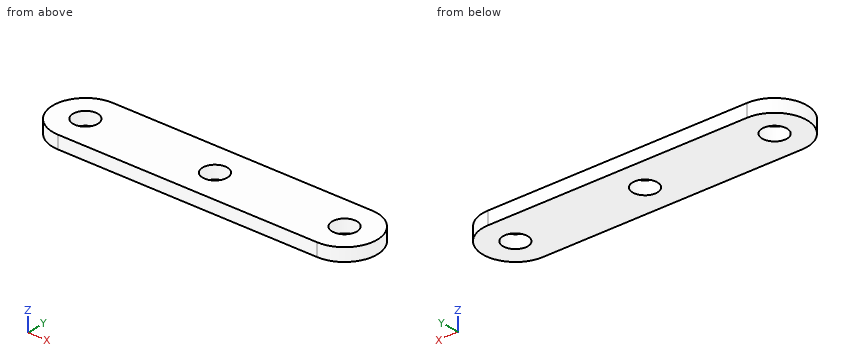
from build123d import *

# Parameters (mm, degrees)
SALIENTE_EXTRUIR1_DEPTH = 1.27
CROQUIS2_R              = 2.413
CORTAR_EXTRUIR1_DEPTH   = 33.478248105
MATRIZL1_COUNT          = 3
MATRIZL1_PITCH          = 25.4


with BuildPart() as part:
    # Croquis1 → Saliente-Extruir1 (new, symmetric)
    with BuildSketch(Plane.XY):
        with BuildLine():
            Line((25.4, -6.35), (-25.4, -6.35))
            ThreePointArc((-25.4, -6.35), (-31.75, 0), (-25.4, 6.35))
            Line((-25.4, 6.35), (25.4, 6.35))
            ThreePointArc((25.4, 6.35), (31.75, 0), (25.4, -6.35))
        make_face()
    extrude(amount=SALIENTE_EXTRUIR1_DEPTH, both=True)

    # Croquis2 → Cortar-Extruir1 (cut, through all)
    with BuildSketch(Plane.XY.offset(1.27)):
        with Locations((-25.4, 0)):
            Circle(CROQUIS2_R)
    cortar_extruir1 = extrude(amount=-CORTAR_EXTRUIR1_DEPTH, mode=Mode.SUBTRACT)

    # MatrizL1: Cortar-Extruir1 ×3
    with Locations(*[(i * MATRIZL1_PITCH, 0, 0) for i in range(1, MATRIZL1_COUNT)]):
        add(cortar_extruir1, mode=Mode.SUBTRACT)


solid = part.part
Source: CAD feature listing. Evaluate the final solid. Frame: model axes, mm. Give positions to 0.01 mm unless a question says otherwise; leave off trailing zeros. Write each loop counter-clockwise with the first axis right and the second up, starting at its lowest first coordinate (ties: lowest second). Pieces come first, ordered by that corner, then holes. Notation, with made-up numbers: (-13, 35) - (1, 35) arc R3 cw to (1, 39) - close; hole circle Ø11 at (28.25, 74.5). An arc over 180 degrees is marked (long way). Write item = value, one per line. Start each with the question number.
Q1. Pin query (flat end, axial travel): pin 1 Ø3 at (x, y) = (25.4, 0) entering from -Z. Return the tip coordinate at first contact, or that it passes through.
Q2. Cut plane C-C, the plane y = -3.5. Return loops of the section in (x, z).
Q3. Material intervals for probe 1 along Y at (x, z) = (0, -0.1); probe 2 along X at (y, z) = (-0.5, -0.6); probe 3 along X at (y, z) = (-0.75, 0.25), sorted ascending.
Q4. Cut plane A-A, the plane y = 0. Return loops of the section in (x, z).
Q5. Cut plane D-D, the plane y = 4. Return loops of the section in (x, z), then the cut area to 3 significant figures.
Q6. Cut plane B-B, the plane x = 0. Return loops of the section in (y, z), then the cut area to 3 significant figures.
Computed values:
q1.pin_1 = through
q2.outline = (-30.7, -1.27) - (30.7, -1.27) - (30.7, 1.27) - (-30.7, 1.27) - close
q3.probe_1 = -6.35 to -2.41, 2.41 to 6.35
q3.probe_2 = -31.73 to -27.76, -23.04 to -2.36, 2.36 to 23.04, 27.76 to 31.73
q3.probe_3 = -31.71 to -27.69, -23.11 to -2.29, 2.29 to 23.11, 27.69 to 31.71
q4.outline = (-31.75, -1.27) - (-27.81, -1.27) - (-27.81, 1.27) - (-31.75, 1.27) - close; (-22.99, -1.27) - (-2.41, -1.27) - (-2.41, 1.27) - (-22.99, 1.27) - close; (2.41, -1.27) - (22.99, -1.27) - (22.99, 1.27) - (2.41, 1.27) - close; (27.81, -1.27) - (31.75, -1.27) - (31.75, 1.27) - (27.81, 1.27) - close
q5.outline = (-30.33, -1.27) - (30.33, -1.27) - (30.33, 1.27) - (-30.33, 1.27) - close
q5.area = 154 mm²
q6.outline = (-6.35, -1.27) - (-2.41, -1.27) - (-2.41, 1.27) - (-6.35, 1.27) - close; (2.41, -1.27) - (6.35, -1.27) - (6.35, 1.27) - (2.41, 1.27) - close
q6.area = 20.0 mm²
